Model file for the job. Use its own axes, mm. Face numbers are marked on the shaded views. Coordinates: 2 decimals unless noted, no trailing zeros. Order: outer loops, then holes, each group sorted by start corner. A loop starts at its lowest first (then second) coordinate and runs counter-clockwise, first axis right, second up. Notation, with made-up numbers: (52.25, -10) -> (111.25, -10) arc R35 ccw to (111.25, 24) -> close; hole circle Ø2 at (-24, 29.25). An arc over 180 degrees is marked (long way). Write item = value, one per line. Start each with the question number.
Q1. Flat gauge pins, fed straight in: pin 1 (2 mm diameter, centred on x = -4.5, y = 1, fed in from -Z); pin 2 (2 mm diameter, centred on y = -13, z = -10.5, fed in from +X); pin 3 (1 mm diameter, centred on x = 4, y = 1.5, fed in from +Z). Where does each tip first touch, or does it go through?
Q2. Cut at C-C, the plane z = 0. List the corners of the cut face in (x, y).
Q3. Cut at D-D, the plane x = 4.75. List the corners of the cut face in (y, z), plus the area to 3 significant figures.
Q4. Mould opens along Z. For the marked faces 1 and 2 say: +Z half, -Z half, draft (parallel to the pull), parting line (faces both ways), or undercut.
Q5. Cut at A-A, the plane z = 9.75. List the corners of the cut face in (x, y), plus the area to 3 significant figures.
Q6. Cut at B-B, the plane y = -4.5. List the corners of the cut face in (x, z).
Q7. Wall check: line 1 (X direction, y = 1.5, z = 0); line 2 (Z direction, x = 0, y = -15.25); line 3 (Y direction, x = -1.75, z = -2.5). Give the ranges that are in metal, low to high. Write a range as from..to.
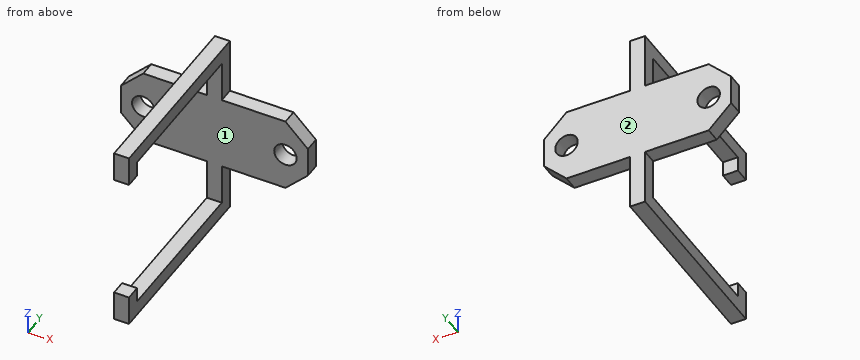
from build123d import *

# Parameters (mm, degrees)
SKETCH_1_W      = 25
SKETCH_1_H      = 10
SKETCH_1_R      = 1.5
EXTRUDE_1_DEPTH = 2
EXTRUDE_3_DEPTH = 1
CHAMFER_1_SIZE  = 3


with BuildPart() as part:
    # 스케치1 → 보스-돌출1 (new body)
    with BuildSketch(Plane(origin=(0, 0, 0), x_dir=(1, 0, 0), z_dir=(0, 1, 0))):
        Rectangle(SKETCH_1_W, SKETCH_1_H)
        with Locations(Location((-9.5, 0, 0), (0, 0, 270))):
            Circle(SKETCH_1_R, mode=Mode.SUBTRACT)
        with Locations(Location((9.5, 0, 0), (0, 0, 270))):
            Circle(SKETCH_1_R, mode=Mode.SUBTRACT)
    extrude(amount=EXTRUDE_1_DEPTH)

    # 스케치4 → 보스-돌출3 (add, symmetric)
    with BuildSketch(Plane(origin=(0, 0, 0), x_dir=(0, 0, -1), z_dir=(1, 0, 0))):
        Polygon((-10.5, 0), (-5, 0), (-5, 2), (-12.5, 2), (-12.5, -23), (-8.5, -23), (-8.5, -21), (-10.5, -21), align=None)
        Polygon((5, 2), (5, 0), (10.5, 0), (10.5, -21), (8.5, -21), (8.5, -23), (12.5, -23), (12.5, 2), align=None)
    extrude(amount=EXTRUDE_3_DEPTH, both=True)

    # 모따기1
    chamfer_1_edges = [part.edges().sort_by_distance(p)[0] for p in [
        (12.5, 1, -5),
        (12.5, 1, 5),
        (-12.5, 1, -5),
        (-12.5, 1, 5),
    ]]
    chamfer(chamfer_1_edges, length=CHAMFER_1_SIZE)


solid = part.part
Here are the results:
q1.pin_1 = -5
q1.pin_2 = 1
q1.pin_3 = 5
q2.outline = (-12.5, 0) -> (-11, 0) -> (-11, 2) -> (-12.5, 2) -> close; (-8, 0) -> (8, 0) -> (8, 2) -> (-8, 2) -> close; (11, 0) -> (12.5, 0) -> (12.5, 2) -> (11, 2) -> close
q3.outline = (0, -5) -> (2, -5) -> (2, 5) -> (0, 5) -> close
q3.area = 20.0 mm²
q4.face_1 = undercut
q4.face_2 = draft
q5.outline = (-1, -23) -> (1, -23) -> (1, -21) -> (-1, -21) -> close; (-1, 0) -> (1, 0) -> (1, 2) -> (-1, 2) -> close
q5.area = 8.00 mm²
q6.outline = (-1, -12.5) -> (1, -12.5) -> (1, -10.5) -> (-1, -10.5) -> close; (-1, 10.5) -> (1, 10.5) -> (1, 12.5) -> (-1, 12.5) -> close
q7.line_1 = -12.5..-11, -8..8, 11..12.5
q7.line_2 = -12.5..-10.5, 10.5..12.5
q7.line_3 = 0..2
